```python
from build123d import *

# Parameters (mm, degrees)
F0_R     = 38.1
F1_DEPTH = 12.7


with BuildPart() as f1:
    # F0 (on Top) → F1 (new body)
    with BuildSketch(Plane.XY):
        Circle(F0_R)
        Polygon((6.35, 25.4), (6.35, 6.35), (25.4, 6.35), (25.4, -6.35), (6.35, -6.35), (6.35, -25.4), (-6.35, -25.4), (-6.35, -6.35), (-25.4, -6.35), (-25.4, 6.35), (-6.35, 6.35), (-6.35, 25.4), align=None, mode=Mode.SUBTRACT)
    extrude(amount=F1_DEPTH)


solid = f1.part
```
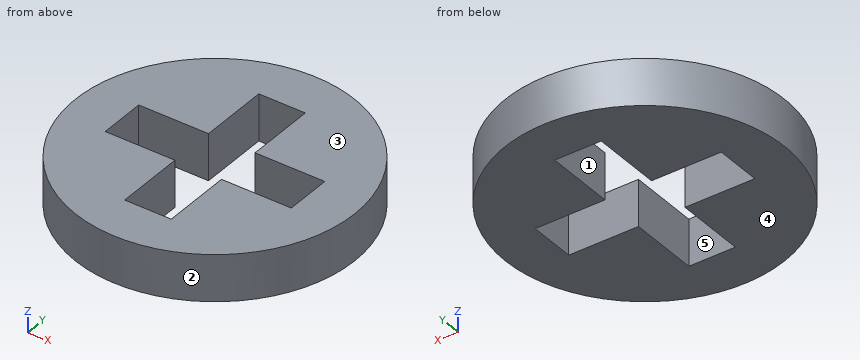
CAD build for the part. Positions are in the model's coordinates, mm. Face numbers are marked on the shaded views. A direction names the side the tool comes from. Give positions to 0.01 mm unless a question says otherwise; leave off trailing zeros. Order: outer loops, then holes, each group sorted by start corner. A loop starts at its lowest first (then second) coordinate and runs counter-clockwise, first axis right, second up.
(1) Saw through at A-A, the plane x = 0. Give the cut face in (y, z), then the cut area to 3 significant figures.
(2) Mould opens along X. For the marked faces 1, 2 and 3 say: released by +X, released by -X, zero draft, split by the parting line, or undercut.
(3) Saw through at B-B, the plane z = 9.5. Give the cut face in (x, y), then the cut area to 3 significant figures.
(4) Flat gauge pins, fed straight in: pin 1 (6.5 mm diameter, centred on x = -19, z = 8.5, fed in from -Y); pin 2 (4 mm diameter, centred on x = 18, z = 6, fed in from +Y); pin 3 (1.5 mm diameter, centred on y = 25, z = 5, fed in from -X). Where does each tip first touch, or does it go through?
(5) Drill centre lines: L1, parallel to Y at x = 21.5, z = 12.25; L2, parallel to X at y = -12, z = 0.5; L3, parallel to X at y = -14, z = 9.25. Where is each one in solid material? Low to high.
(6) Saw through at D-D, the plane y = -31. Give the cut face in (x, z), then the cut area to 3 significant figures.
(7) Tool access for the marked faces 4 and 5: list every direction of +Z, -Z, +X, -X, +Y, -Y with a clear straight run to the whole face (end or side of a thin tool).
Results found:
1. outline: (-38.1, 0) - (-25.4, 0) - (-25.4, 12.7) - (-38.1, 12.7) - close; (25.4, 0) - (38.1, 0) - (38.1, 12.7) - (25.4, 12.7) - close
1. area: 323 mm2
2. face 1: undercut
2. face 2: split by the parting line
2. face 3: zero draft
3. outline: circle Ø76.2 at (0, 0); hole (-25.4, -6.35) - (-6.35, -6.35) - (-6.35, -25.4) - (6.35, -25.4) - (6.35, -6.35) - (25.4, -6.35) - (25.4, 6.35) - (6.35, 6.35) - (6.35, 25.4) - (-6.35, 25.4) - (-6.35, 6.35) - (-25.4, 6.35) - close
3. area: 3,430 mm2
4. pin 1: stops at y = -34.69
4. pin 2: stops at y = 34.58
4. pin 3: stops at x = -29.39
5. L1: y = -31.45 to -6.35, 6.35 to 31.45
5. L2: x = -36.16 to -6.35, 6.35 to 36.16
5. L3: x = -35.43 to -6.35, 6.35 to 35.43
6. outline: (-22.15, 0) - (22.15, 0) - (22.15, 12.7) - (-22.15, 12.7) - close
6. area: 563 mm2
7. face 4: -Z, +X, -X, +Y, -Y
7. face 5: +Z, -Z
